```python
from build123d import *

# Parameters (mm, degrees)
BOSS_EXTRUDE1_DEPTH = 184.15
SKETCH2_R           = 7.332348419
SKETCH2_R_2         = 6.35
CUT_EXTRUDE1_DEPTH  = 11.1125
SKETCH3_W           = 0.889
SKETCH3_H           = 0.4064
SKETCH3_H_2         = 3.038077808
CHAMFER1_SIZE       = 0.635


with BuildPart() as part:
    # Sketch1 → Boss-Extrude1 (new body)
    with BuildSketch(Plane.XY):
        Polygon((0, 7.332348419), (-6.35, 3.666174209), (-6.35, -3.666174209), (0, -7.332348419), (6.35, -3.666174209), (6.35, 3.666174209), align=None)
    extrude(amount=BOSS_EXTRUDE1_DEPTH)

    # Sketch2 → Cut-Extrude1 (cut)
    with BuildSketch(Plane.XY.offset(184.15)):
        Circle(SKETCH2_R)
        Circle(SKETCH2_R_2, mode=Mode.SUBTRACT)
    extrude(amount=-CUT_EXTRUDE1_DEPTH, mode=Mode.SUBTRACT)

    # Sketch3 → Cut-Revolve1 (revolve, cut)
    with BuildSketch(Plane(origin=(0, 0, 0), x_dir=(0, 0, -1), z_dir=(1, 0, 0)), mode=Mode.PRIVATE) as cut_revolve1_sk:
        with Locations((-181.4195, 6.1468)):
            Rectangle(SKETCH3_W, SKETCH3_H)
        with Locations((-97.9805, 7.462638904)):
            Rectangle(SKETCH3_W, SKETCH3_H_2)
    revolve(cut_revolve1_sk.sketch.rotate(Axis((0, 0, 184.15), (0, 0, -1)), 90), axis=Axis((0, 0, 184.15), (0, 0, -1)), mode=Mode.SUBTRACT)

    # Chamfer1
    chamfer1_edges = [part.edges().sort_by_distance(p)[0] for p in [
        (-6.35, 0, 184.15),
    ]]
    chamfer(chamfer1_edges, length=CHAMFER1_SIZE)


solid = part.part
```
Here's how the part is built. I have some questions about the finished solid (model axes, mm). A direction names the side the tool comes from. Coordinates: 2 decimals unless noted, no trailing zeros. Order: outer loops, then holes, each group sorted by start corner. A loop starts at its lowest first (then second) coordinate and runs counter-clockwise, first axis right, second up. Notation, with made-up numbers: M -9.5,19 L 44.5,19 A12 cw 44.5,36 Z; hole C 72.5,46 d9. An arc over 180 degrees is marked long. Answer as a JSON object with one key per item and string values. Group by question number.
(1) Which directions (+Z, -Z, +X, -X, +Y, -Y) give clear straight access to the entire face, cutting with the end or side of a thin tool? Please do faces 1 (the face through (-1.38, -6.2, 177.06)), 2 (the face through (6, -3, 173.038)), 3 (the face through (6, 3, 173.038)), 4 (the face through (-6, 3, 173.038)).
(2) If we mould it in two halves opening along Z, with no side actions, what happens to faces 5 (the face through (-1.38, -6.2, 182.7)), 6 (the face through (5, -4, 97.536)), 7 (the face through (0, 0, 184.15)), 8 (the face through (5.669, -1.785, 97.974))? For each: released by +Z, released by -Z, zero draft, split by the parting line, or undercut.
(3) I need wall thicknesses on probe 1 along Z at (x, y) = (2.75, 5.5) (3 decimals); probe 2 along X at (y, z) = (-5.5, 87); probe 3 along Y at (x, z) = (-1.75, 157.5). Which ranges of each line are inside material? Lowest first, please.
(4) For pin 1 (0.9 mm diameter, centred on x = 1, y = -6.5, fed in from +Z); pin 2 (0.9 mm diameter, centred on x = 0, y = 6.5, fed in from +Z) (3 decimals); pin 3 (2 mm diameter, centred on x = -3, z = 117.5, fed in from +Y), each with a flat end and sliding along its axis, tell me the tip position at first contact or that it passes through.
(5) Suppose I cut it at A-A, the plane z = 16.5. Please give me the cut outline in (x, y).
Values found:
{
 "1": {"face 1": "+Z", "face 2": "+Z, +X, -Y", "face 3": "+Z, +X, +Y", "face 4": "+Z, -X, +Y"},
 "2": {"face 5": "zero draft", "face 6": "undercut", "face 7": "released by +Z", "face 8": "undercut"},
 "3": {"probe 1": "z = 0 to 97.536, 98.425 to 180.975, 181.864 to 183.716", "probe 2": "x = -3.17 to 3.17", "probe 3": "y = -6.32 to 6.32"},
 "4": {"pin 1": "stops at z = 183.74", "pin 2": "stops at z = 183.815", "pin 3": "stops at y = 6.18"},
 "5": {"outline": "M -6.35,-3.67 L 0,-7.33 L 6.35,-3.67 L 6.35,3.67 L 0,7.33 L -6.35,3.67 Z"}
}
